from build123d import *

# Parameters (mm, degrees)
F0_R     = 609.6
F0_R_2   = 6.35
F0_R_3   = 25.4
F1_DEPTH = 19.05
F2_R     = 152.4
F2_R_2   = 142.875
F3_DEPTH = 12.7


with BuildPart() as f1:
    # F0 (on Front) → F1 (new body, symmetric)
    with BuildSketch(Plane.XZ):
        Circle(F0_R)
        with Locations((0, -50.8)):
            Circle(F0_R_2, mode=Mode.SUBTRACT)
        with Locations((-50.8, 0)):
            Circle(F0_R_2, mode=Mode.SUBTRACT)
        Circle(F0_R_3, mode=Mode.SUBTRACT)
        with Locations((50.8, 0)):
            Circle(F0_R_2, mode=Mode.SUBTRACT)
        with Locations((0, 50.8)):
            Circle(F0_R_2, mode=Mode.SUBTRACT)
    extrude(amount=F1_DEPTH, both=True)

    # F2 (on face) → F3 (cut)
    with BuildSketch(Plane.XZ.offset(19.05)):
        Circle(F2_R)
        Circle(F2_R_2, mode=Mode.SUBTRACT)
    extrude(amount=-F3_DEPTH, mode=Mode.SUBTRACT)


solid = f1.part
CAD build for the part. Positions are in the model's coordinates, mm. A direction names the side the tool comes from. Round coordinates to 2 decimals unless told otherwise and drop trailing zeros. Write each loop counter-clockwise with the first axis right and the second up, starting at its lowest first coordinate (ties: lowest second). Pieces come first, ordered by that corner, then holes. Notation, with made-up numbers: (-7, 66) -> (23, 66) arc R10 ccw to (23, 81) -> close; hole circle Ø6 at (12, -22.5). An arc over 180 degrees is marked (long way). Answer as a JSON object with one key per item and string values.
(1) Band-saw the part on C-C, the plane z = 347.5. List the corners of the cut face in (x, y), then the cut area to 3 significant figures.
Reported:
{"outline": "(-500.86, -19.05) -> (500.86, -19.05) -> (500.86, 19.05) -> (-500.86, 19.05) -> close", "area": "38,200 mm^2"}
(2) Band-saw the part on D-D, the plane x = 396.5. List the corners of the cut face in (y, z).
Reported:
{"outline": "(-19.05, -463.03) -> (19.05, -463.03) -> (19.05, 463.03) -> (-19.05, 463.03) -> close"}
(3) Two-plate mould, pull along Z, no slides. Class faces 3 (the face through (-2, -19.05, -30)), 4 (the face through (-483.76, -0.27, -370.93)), 5 (the face through (-142.737, -12.789, 6.282)): +Z half, -Z half, draft (parallel to the pull), parting line (faces both ways), or undercut.
Reported:
{"face 3": "draft", "face 4": "parting line", "face 5": "undercut"}
(4) Band-saw the part on A-A, the plane y = 6.5. List the corners of the cut face in (x, z), then the cut area to 3 significant figures.
Reported:
{"outline": "circle Ø1219.2 at (0, 0); hole circle Ø12.7 at (-50.8, 0); hole circle Ø50.8 at (0, 0); hole circle Ø12.7 at (0, -50.8); hole circle Ø12.7 at (0, 50.8); hole circle Ø12.7 at (50.8, 0)", "area": "1,160,000 mm^2"}
(5) Probe probe 1 along Z at (x, y) = (0, -7) (3 decimals); probe 2 along Z at (x, y) = (0, -3); probe 3 along Z at (x, y) = (-56, -12.5). List the from-to ranges inside material, lowest first. Write a range as [from, to].
Reported:
{"probe 1": "z = [-609.6, -152.4], [-142.875, -57.15], [-44.45, -25.4], [25.4, 44.45], [57.15, 142.875], [152.4, 609.6]", "probe 2": "z = [-609.6, -57.15], [-44.45, -25.4], [25.4, 44.45], [57.15, 609.6]", "probe 3": "z = [-607.02, -141.74], [-131.44, -3.64], [3.64, 131.44], [141.74, 607.02]"}
(6) Pin check, flat tips, straight feed: P1, Ø4, axis at x = 151.5, y = 0, coming from the -Z side; P2, Ø11.5, axis at x = 0, z = -50.8, coming from the -Y side; P3, Ø12, axis at x = -474, y = -12.5, coming from the +Z side; P4, Ø10, axis at x = 232.5, y = -6.5, coming from the +Z side. Stop position of each tip, or through.
Reported:
{"P1": "stops at z = -590.98", "P2": "passes through", "P3": "stops at z = 390.63", "P4": "stops at z = 565.56"}
(7) Band-saw the part on B-B, the plane x = -115.5. List the corners of the cut face in (y, z), then the cut area to 3 significant figures.
Reported:
{"outline": "(-19.05, -598.56) -> (19.05, -598.56) -> (19.05, 598.56) -> (-19.05, 598.56) -> (-19.05, 99.43) -> (-6.35, 99.43) -> (-6.35, 84.1) -> (-19.05, 84.1) -> (-19.05, -84.1) -> (-6.35, -84.1) -> (-6.35, -99.43) -> (-19.05, -99.43) -> close", "area": "45,200 mm^2"}
(8) Which spindle directions (+Z, -Z, +X, -X, +Y, -Y) get a long thin tool onto all of the face, cutting with end or side? Do faces 1 (the face through (-5.506, 0.267, -24.796)), 2 (the face through (44.4, -6.35, 136.2)). Say none if no direction does.
Reported:
{"face 1": "+Y, -Y", "face 2": "-Y"}
